```python
from build123d import *
from build123d.topology import SkipClean

# Parameters (mm, degrees)
MAIN_DEPTH            = 2
ESQUISSE2_R           = 2.5
ORIGINALBRACKET_DEPTH = 1
ESQUISSE3_R           = 1.3
FIXINGHOLE_DEPTH      = 26.773047938


with BuildPart() as part:
    # Esquisse1 → Main (new body)
    with BuildSketch(Plane.XY):
        with BuildLine():
            Line((0.625, 5.464373249), (22.340909091, 2.980567227))
            ThreePointArc((22.340909091, 2.980567227), (25, 0), (22.340909091, -2.980567227))
            Line((22.340909091, -2.980567227), (0.625, -5.464373249))
            ThreePointArc((0.625, -5.464373249), (-5.5, 0), (0.625, 5.464373249))
        make_face()
        with BuildLine():
            Line((0.336544343, 3.534011588), (16.539602446, 1.990992444))
            ThreePointArc((16.539602446, 1.990992444), (18.35, 0), (16.539602446, -1.990992444))
            Line((16.539602446, -1.990992444), (0.336544343, -3.534011588))
            ThreePointArc((0.336544343, -3.534011588), (-3.55, 0), (0.336544343, 3.534011588))
        make_face(mode=Mode.SUBTRACT)
    extrude(amount=MAIN_DEPTH)

    # Esquisse2 → OriginalBracket (add)
    with SkipClean():  # the faces are left unmerged after this step: merging them gives an invalid solid
        with BuildSketch(Plane(origin=(0, 0, 0), x_dir=(-1, 0, 0), z_dir=(0, 0, -1))):
            with BuildLine():
                Line((-0.625, -5.464373249), (-22.340909091, -2.980567227))
                ThreePointArc((-22.340909091, -2.980567227), (-25, 0), (-22.340909091, 2.980567227))
                Line((-22.340909091, 2.980567227), (-0.625, 5.464373249))
                ThreePointArc((-0.625, 5.464373249), (5.5, 0), (-0.625, -5.464373249))
            make_face()
            Circle(ESQUISSE2_R, mode=Mode.SUBTRACT)
        extrude(amount=ORIGINALBRACKET_DEPTH)

    # Esquisse3 → FixingHole (cut, through all)
    with SkipClean():  # the faces are left unmerged after this step: merging them gives an invalid solid
        with BuildSketch(Plane.XY.offset(2)):
            with Locations((22, 0)):
                Circle(ESQUISSE3_R)
        extrude(amount=-FIXINGHOLE_DEPTH, mode=Mode.SUBTRACT)


solid = part.part
```
Work out the finished part from the listing and answer in its coordinate system (mm). A direction names the side the tool comes from. Round coordinates to 2 decimals unless told otherwise and drop trailing zeros. Write each loop counter-clockwise with the first axis right and the second up, starting at its lowest first coordinate (ties: lowest second). Pieces come first, ordered by that corner, then holes. Notation, with made-up numbers: (72, -27.5) - (100, -27.5) arc R31 cw to (100, -1.5) - close; hole circle Ø4 at (33.5, 14). An arc over 180 degrees is marked (long way). Return JSON: item names as keys, results as strings. Group by question number.
Q1. For faces 3 (the flat face through (8.55, -2.75, 0.99)), 4 (the flat face through (10, 0, -1)), determine the directions among +Z, -Z, +X, -X, +Y, -Y from which every point of the face is accessible in a straight line to the end or side of a thin tool.
Q2. Find the intervals of material crossed by L1, parallel to Y at x = 0, z = 1.4; L2, parallel to Z at x = 10.5, y = -1.5; L3, parallel to X at y = 2, z = -0.75, in increasing order.
Q3. The part is cut by section C-C on z = 0.45. Write down the section's boundary in (x, y) (3 decimals), then the cut area to 3 significant figures.
Q4. The part is cut by section B-B on x = 0. Write down the section's boundary in (y, z).
Q5. Each of these flat-tipped pins is pushed along its axis until it touches: pin 1 Ø3.5 at (x, y) = (2.5, -1.5) entering from +Z; pin 2 Ø1 at (x, z) = (8, 1.5) entering from -Y; pin 3 Ø4.5 at (x, y) = (0, 0) entering from +Z. Where does it stop, or does it pass through?
Q6. The part is cut by section A-A on y = 0. Write down the section's boundary in (x, z), then the cut area to 3 significant figures.
Q7. The mould has two halves that part along Y. Classify faces 1 (the flat face through (10, -4, 2)), 2 (the flat face through (8.325, 2.773, 0.986)): released by +Y, released by -Y, zero draft, split by the parting line, or undercut.
Q8. The part is cut by section D-D on x = 15.5. Write down the section's boundary in (y, z).
Solved:
{
 "1": {"face 3": "+Z", "face 4": "-Z, +X, -X, +Y, -Y"},
 "2": {"L1": "-5.5 to -3.55, 3.55 to 5.5", "L2": "-1 to 0", "L3": "-5.12 to -1.5, 1.5 to 24.24"},
 "3": {"outline": "(0.625, -5.464) - (22.341, -2.981) arc R3 ccw to (22.341, 2.981) - (0.625, 5.464) arc R5.5 ccw (long way) to start; hole (0.337, -3.534) - (16.54, -1.991) arc R2 ccw to (16.54, 1.991) - (0.337, 3.534) arc R3.55 ccw (long way) to start; hole circle Ø2.6 at (22, 0)", "area": "127 mm²"},
 "4": {"outline": "(-5.5, -1) - (-2.5, -1) - (-2.5, 0) - (-3.55, 0) - (-3.55, 2) - (-5.5, 2) - close; (2.5, -1) - (5.5, -1) - (5.5, 2) - (3.55, 2) - (3.55, 0) - (2.5, 0) - close"},
 "5": {"pin 1": "z = 0", "pin 2": "y = -4.68", "pin 3": "through"},
 "6": {"outline": "(-5.5, -1) - (-2.5, -1) - (-2.5, 0) - (-3.55, 0) - (-3.55, 2) - (-5.5, 2) - close; (2.5, -1) - (20.7, -1) - (20.7, 2) - (18.35, 2) - (18.35, 0) - (2.5, 0) - close; (23.3, -1) - (25, -1) - (25, 2) - (23.3, 2) - close", "area": "34.9 mm²"},
 "7": {"face 1": "zero draft", "face 2": "undercut"},
 "8": {"outline": "(-3.76, -1) - (3.76, -1) - (3.76, 2) - (2.09, 2) - (2.09, 0) - (-2.09, 0) - (-2.09, 2) - (-3.76, 2) - close"}
}
